```python
from build123d import *

# Parameters (mm, degrees)
SKETCH1_R           = 4
BOSS_EXTRUDE2_DEPTH = 5
FILLET3_R           = 3


with BuildPart() as part:
    # Sketch1 → Boss-Extrude2 (new body)
    with BuildSketch(Plane.XY):
        with BuildLine():
            ThreePointArc((-2.823470485, 6.805503827), (0, 7.367962264), (2.823470485, 6.805503827))
            Line((2.823470485, 6.805503827), (12.934326877, 2.610707185))
            ThreePointArc((12.934326877, 2.610707185), (14.507189087, 2.140514293), (16.142912091, 2.001276593))
            Line((16.142912091, 2.001276593), (56.478756137, 2.721951573))
            Line((56.478756137, 2.721951573), (56.478756137, 7.377996322))
            ThreePointArc((56.478756137, 7.377996322), (0, 21.5), (-56.478756137, 7.377996322))
            Line((-56.478756137, 7.377996322), (-56.478756137, 2.721951573))
            Line((-56.478756137, 2.721951573), (-16.142912091, 2.001276593))
            ThreePointArc((-16.142912091, 2.001276593), (-14.507189087, 2.140514293), (-12.934326877, 2.610707185))
            Line((-12.934326877, 2.610707185), (-2.823470485, 6.805503827))
        make_face()
        with Locations((-16, 10)):
            Circle(SKETCH1_R, mode=Mode.SUBTRACT)
        with Locations((16, 10)):
            Circle(SKETCH1_R, mode=Mode.SUBTRACT)
    extrude(amount=BOSS_EXTRUDE2_DEPTH)

    # Fillet3
    # the kernel refuses this fillet: 3 mm, written as the material it takes off along each edge
    with BuildSketch(Plane(origin=(56.478756137, 2.721951573, -7.367195529), x_dir=(-0.9998404258161971, -0.017864011410817362, 0), z_dir=(0, 0, 1)), Plane(origin=(-56.478756137, 2.721951573, -7.367195529), x_dir=(0, 1, 0), z_dir=(0, 0, 1))) as fillet3_piece_1:
        with BuildLine():
            CenterArc((FILLET3_R * 0.982292737151, -FILLET3_R), FILLET3_R, 90, 88.976413094)
            Line((-FILLET3_R * 0.0175476886652, -FILLET3_R * 0.982135988589), (0, 0))
            Line((0, 0), (FILLET3_R * 0.982292737151, 0))
        make_face()
    extrude(amount=19.734391057, mode=Mode.SUBTRACT)
    with BuildSketch(Plane(origin=(56.478756137, 7.377996322, -4.596333569), x_dir=(0, -1, 0), z_dir=(0, 0, 1))) as fillet3_piece_2:
        with BuildLine():
            CenterArc((1.8154063, -3), FILLET3_R, 90, 62.800936738)
            ThreePointArc((-0.852865239, -1.628749843), (-0.429551947, -0.812741542), (0, 0))
            Line((0, 0), (1.8154063, 0))
        make_face()
    extrude(amount=14.192667139, mode=Mode.SUBTRACT)
    with BuildSketch(Plane(origin=(-56.478756137, 7.377996322, -4.596333569), x_dir=(0, -1, 0), z_dir=(0, 0, 1))) as fillet3_piece_3:
        with BuildLine():
            CenterArc((1.8154063, 3), FILLET3_R, 207.199063262, 62.800936738)
            ThreePointArc((-0.852865239, 1.628749843), (-0.429551947, 0.812741542), (0, 0))
            Line((0, 0), (1.8154063, 0))
        make_face()
    extrude(amount=14.192667139, mode=Mode.SUBTRACT)


solid = part.part
```
Model file for the job. Use its own axes, mm. A direction names the side the tool comes from. Coordinates: 2 decimals unless noted, no trailing zeros. Order: outer loops, then holes, each group sorted by start corner. A loop starts at its lowest first (then second) coordinate and runs counter-clockwise, first axis right, second up. Notation, with made-up numbers: (40, -21.5) - (64, -21.5) arc R21 cw to (64, -0.5) - close; hole circle Ø3 at (53.25, -19.5). An arc over 180 degrees is marked (long way). Return JSON: item names as keys, results as strings. Group by question number.
1) Mould opens along Y. For faces 3 (the cylindrical face through (56.037, 7.129, 2.465)), 4 (the flat face through (7.808, 4.737, 2.465)), 5 (the cylindrical face through (-20, 10, 2)) say: released by +Y, released by -Y, zero draft, split by the parting line, or undercut.
2) Saw through at A-A, the plane z = 3.65. Write the cut outline in (x, y).
3) Saw through at C-C, the plane y = 10. Write the cut outline in (x, z), plus the area to 3 significant figures.
4) Tool access for faces 1 (the flat face through (-1, 10, 0)), 2 (the flat face through (-7.9, 4.7, 2.5)): list every direction of +Z, -Z, +X, -X, +Y, -Y with a clear straight run to the whole face (end or side of a thin tool).
5) Saw through at B-B, the plane x = 15. Write the cut outline in (y, z).
6) Probe line 1 (X direction, y = 12.75, z = 4.05); line 2 (X direction, y = 10.25, z = 3.5); line 3 (Y direction, x = -0.5, z = 3.8). List the from-to ranges inside material, lowest first. Write a range as from..to.
7) Saw through at D-D, the plane x = 43.5. Write the cut outline in (y, z).
8) Flat gauge pins, fed straight in: P1, Ø2, axis at x = -16.5, y = 6.5, coming from the +Z side; P2, Ø5, axis at x = -16, y = 10, coming from the +Z side. Where does each tip first touch, or does it go through?
Values found:
{
 "1": {"face 3": "released by +Y", "face 4": "released by -Y", "face 5": "undercut"},
 "2": {"outline": "(-56.48, 5.62) arc R3 ccw to (-53.53, 2.67) - (-16.14, 2) arc R8 ccw to (-12.93, 2.61) - (-2.82, 6.81) arc R7.37 cw to (2.82, 6.81) - (12.93, 2.61) arc R8 ccw to (16.14, 2) - (53.53, 2.67) arc R3 ccw to (56.48, 5.62) arc R3 ccw to (54.85, 8.23) arc R120 ccw to (-54.85, 8.23) arc R3 ccw to start; hole circle Ø8 at (-16, 10); hole circle Ø8 at (16, 10)"},
 "3": {"outline": "(-51.26, 0) - (-20, 0) - (-20, 5) - (-51.26, 5) - close; (-12, 0) - (12, 0) - (12, 5) - (-12, 5) - close; (20, 0) - (51.26, 0) - (51.26, 5) - (20, 5) - close", "area": "433 mm²"},
 "4": {"face 1": "-Z, +X, -X, +Y, -Y", "face 2": "+Z, -Z, -Y"},
 "5": {"outline": "(2.06, 0) - (6.13, 0) - (6.13, 5) - (2.06, 5) - close; (13.87, 0) - (20.56, 0) - (20.56, 5) - (13.87, 5) - close"},
 "6": {"line 1": "x = -44.98..-18.9, -13.1..13.1, 18.9..44.98", "line 2": "x = -50.73..-19.99, -12.01..12.01, 19.99..50.73", "line 3": "y = 7.35..21.5"},
 "7": {"outline": "(2.49, 0) - (13.34, 0) - (13.34, 5) - (2.49, 5) - close"},
 "8": {"P1": "stops at z = 5", "P2": "passes through"}
}
